Input: part model. Units: mm. Frame: model coordinates. Round coordinates to 2 decimals unless told otherwise and drop trailing zeros. Write each loop counter-clockwise with the first axis right and the second up, starting at its lowest first coordinate (ties: lowest second). Pieces come first, ordered by that corner, then holes. Notation, with made-up numbers: (-9, 86) - (34, 86) arc R14 cw to (34, 93) - close; hole circle Ø3 at (-37, -24). An arc over 180 degrees is marked (long way). Use one line per item in the form item = value.
```python
from build123d import *

# Parameters (mm, degrees)
F1_DEPTH = 3


with BuildPart() as f1:
    # F0 (on Front) → F1 (new body)
    with BuildSketch(Plane.XZ):
        with BuildLine():
            ThreePointArc((-9.319805, 31.819805), (-19.074579, 17.220754), (-22.5, 0))
            ThreePointArc((-22.5, 0), (-1.209572, -22.467464), (22.36995, -2.415646))
            ThreePointArc((22.36995, -2.415646), (22.434928, 0), (22.36995, 2.415646))
            ThreePointArc((22.36995, 2.415646), (18.847563, 17.593372), (10.353786, 30.655774))
            ThreePointArc((10.353786, 30.655774), (9.273792, 31.773792), (8.155774, 32.853786))
            ThreePointArc((8.155774, 32.853786), (-0.778474, 35.657185), (-9.319805, 31.819805))
        make_face()
        with BuildLine():
            ThreePointArc((22.36995, 2.415646), (22.434928, 0), (22.36995, -2.415646))
            ThreePointArc((22.36995, -2.415646), (22.5, 0), (22.36995, 2.415646))
        make_face()
        with BuildLine():
            ThreePointArc((10.353786, 30.655774), (9.319805, 31.819805), (8.155774, 32.853786))
            ThreePointArc((8.155774, 32.853786), (9.273792, 31.773792), (10.353786, 30.655774))
        make_face()
    extrude(amount=F1_DEPTH)


solid = f1.part
```
(1) Cut plane A-A on y = -0.55. Output: boundary loops of the cut face in (x, z).
Derived:
outline = (-22.5, 0) arc R22.5 ccw to (22.37, -2.42) arc R22.5 ccw to (22.37, 2.42) arc R44.93 ccw to (10.35, 30.66) arc R13.18 ccw to (8.16, 32.85) arc R13.18 ccw to (-9.32, 31.82) arc R45 ccw to start
(2) Cut plane C-C on z = -16.5. Output: boundary loops of the cut face in (x, y).
Derived:
outline = (-15.3, -3) - (15.3, -3) - (15.3, 0) - (-15.3, 0) - close
(3) Material intervals for L1, parallel to Z at x = 14, y = -2.1; L2, parallel to Z at x = 18.5, y = -0.75; L3, parallel to X at y = -1.75, z = -10, sorted ascending.
Derived:
L1 = -17.61 to 26.21
L2 = -12.81 to 18.39
L3 = -20.16 to 20.16
(4) Cut plane B-B on x = 16. Output: boundary loops of the cut face in (y, z), then the cut area to 3 significant figures.
Derived:
outline = (-3, -15.82) - (0, -15.82) - (0, 23.17) - (-3, 23.17) - close
area = 117 mm^2
(5) First-contact query: pin 1 Ø1.5 at (y, z) = (-1.5, -14.5) entering from -X; pin 2 Ø1.5 at (y, z) = (-1.5, 9) entering from -X. Flat tips, straight axial feed; report the tip coordinate or a pass-through.
Derived:
pin_1 = -17.81
pin_2 = -21.74
